Design review of the part built by this model. Coordinates are the model's own, in mm. Face numbers are marked on the shaded views. A direction names the side the tool comes from. Coordinates: 2 decimals unless noted, no trailing zeros. Write each loop counter-clockwise with the first axis right and the second up, starting at its lowest first coordinate (ties: lowest second). Pieces come first, ordered by that corner, then holes. Notation, with made-up numbers: (61.25, -3.5) -> (110.25, -3.5) arc R27 ccw to (110.25, 17.5) -> close; hole circle Ø5 at (-24.75, -34.75). An arc over 180 degrees is marked (long way). Answer in a Markdown table with one row per item. Add a question column.
Item 1: Clearance check with flat-ended pins moving along their axes: P1, Ø12, axis at x = 18.5, y = -9.5, coming from the -Z side; P2, Ø8, axis at x = 15.5, z = 12.5, coming from the -Y side; P3, Ø6.5, axis at x = -19.5, y = -6, coming from the +Z side; P4, Ø12, axis at x = -2, y = -7.5, coming from the -Z side. State where each tip first meets the part, or that it passes through.
Item 2: Draft analysis for pull direction X (two halves, no side actions). For the marked faces 5, 6 and 7, state which applies: released by +X, released by -X, zero draft, split by the parting line, or undercut.
Item 3: For the marked faces 1, 2, 3 and 4, list the 3-axis set-ups (+Z, -Z, +X, -X, +Y, -Y) from which the entire face can be reached by the end or side of a thin tool; tool diameter is ignored.
Item 4: Take a section at D-D, the plane z = 20. Write out the cut boundary in (x, y), and give its area (3 significant figures).
Item 5: To check wall thickness, follow line 1 (Z direction, x = 17, y = -8.5); line 2 (X direction, y = -5.5, z = -15); line 3 (X direction, y = -13.5, z = -16). State the ranges of each line that lie inside material, in increasing order.
Item 6: Take a section at C-C, the plane z = -15.5. Write out the cut boundary in (x, y), and give its area (3 significant figures).
Item 7: Take a section at A-A, the plane y = -14. Write out the cut boundary in (x, z).
Item 8: Take a section at B-B, the plane y = -7.5. Give the number of separate pieces and of enclosed holes in the cut face, and give its area (3 significant figures).
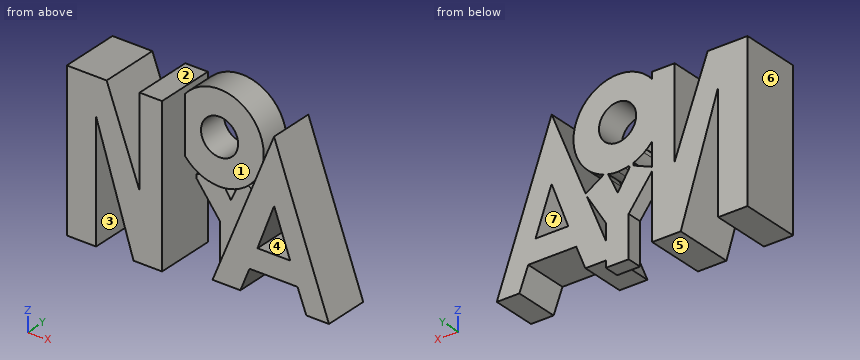
from build123d import *

# Parameters (mm, degrees)
F6_DEPTH  = 20
F7_DEPTH  = 5
F2_R      = 14.8981709713
F8_DEPTH  = 10
F9_DEPTH  = 15
F5_R      = 6.2195311323
F10_DEPTH = 20.001


with BuildPart() as f6:
    # F1 (on Front) → F6 (new body)
    with BuildSketch(Plane.XZ):
        Polygon((-29.4090751559, 23.7889681011), (-29.4090751559, -28.2321553677), (-19.5761136711, -28.2358180233), (-19.5761136711, 11.5612922236), (-7.0128426887, -28.2359085977), (2.5514548179, -28.2359085977), (2.5514548179, 23.8814018667), (-4.9865087494, 23.8814018667), (-4.9865087494, -6.1893938109), (-16.0414669663, 23.7889681011), align=None)
    extrude(amount=F6_DEPTH)



with BuildPart() as f7:
    # F3 (on Front) → F7 (new body)
    with BuildSketch(Plane.XZ):
        Polygon((10.5204042047, -2.2638426162), (8.7501741946, -1.767860345), (8.7501741946, -2.6882454621), (2.6086692233, -5.1982523873), (2.6086692233, -6.4965714701), (10.4526793584, -16.883123666), (10.4526793584, -30.7555552572), (18.1284062564, -30.7555552572), (18.1284062564, -16.9692430645), (24.9908941437, -5.8241511643), (18.8475046307, -2.0414155442), (18.2504130668, -1.177824098), (17.1879893938, -1.9123892853), (17.4144990742, -2.239997033), (14.0946339816, -9.1059375554), (10.1119214669, -2.7744469699), align=None)
    extrude(amount=F7_DEPTH)


with BuildPart() as f6_1:
    add(f6.part)

    add(f7.part)  # F8 merges F7
    # F2 (on Front) → F8 (join)
    with BuildSketch(Plane.XZ):
        with Locations((14.0610327944, 12.1286660433)):
            Circle(F2_R)
    extrude(amount=F8_DEPTH)

    # F4 (on Front) → F9 (join)
    with BuildSketch(Plane.XZ):
        Polygon((54.6711832285, -28.5867527127), (36.2575501204, 22.3937444389), (15.6466114905, -28.5145416856), (24.9638519287, -28.5145416856), (28.0255712569, -20.860247314), (44.1284738481, -20.860247314), (47.089099884, -28.5867527127), align=None)
    extrude(amount=F9_DEPTH)

    # F5 (on Front) + F0 (on Front) → F10 (cut, through all)
    with BuildSketch(Plane.XZ):
        Polygon((10.4725992623, -2.2513235357), (10.0927506823, -2.7248826654), (14.1619760543, -9.0967444703), (17.3306893557, -2.3522656411), (16.3500196487, -2.7850975748), (14.0968551859, -2.7850975748), (11.5571627393, -2.5246159639), align=None)
        with Locations((14.1619760543, 12.4046513811)):
            Circle(F5_R)
        Polygon((4.5241662301, 0.7314007962), (4.2605670169, 0.7808398308), (4.2605670169, -4.4249454513), (8.7323186063, -2.633718365), (8.7323186063, -1.8077495305), (7.9755438492, -1.6129313735), (6.1521744356, -0.636126264), align=None)
    with BuildSketch(Plane.XZ):
        Polygon((30.7015124708, -13.6729935011), (41.6589528322, -13.6729935011), (36.2836048007, 1.1847094047), align=None)
    extrude(amount=F10_DEPTH, mode=Mode.SUBTRACT)


solid = f6_1.part
Answers:
| question | item | result |
|---|---|---|
| 1 | P1 | stops at z = -30.76 |
| 1 | P2 | passes through |
| 1 | P3 | stops at z = 23.79 |
| 1 | P4 | stops at z = -28.24 |
| 2 | face 5 | zero draft |
| 2 | face 6 | released by -X |
| 2 | face 7 | undercut |
| 3 | face 1 | +Z, -Y |
| 3 | face 2 | +Z, -X, +Y, -Y |
| 3 | face 3 | -Z, +Y, -Y |
| 3 | face 4 | +Y, -Y |
| 4 | outline | (-29.41, -20) -> (-14.64, -20) -> (-14.64, 0) -> (-29.41, 0) -> close; (-4.99, -20) -> (2.55, -20) -> (2.55, -10) -> (26.71, -10) -> (26.71, 0) -> (-4.99, 0) -> close; (35.29, -15) -> (37.12, -15) -> (37.12, 0) -> (35.29, 0) -> close |
| 4 | area | 715 mm^2 |
| 5 | line 1 | z = -28.51 to -25.17, -2.48 to 6.87, 17.94 to 26.73 |
| 5 | line 2 | x = -29.41 to -19.58, -11.19 to 2.55, 21.12 to 49.76 |
| 5 | line 3 | x = -29.41 to -19.58, -10.88 to 2.55, 20.71 to 50.12 |
| 6 | outline | (-29.41, -20) -> (-19.58, -20) -> (-19.58, 0) -> (-29.41, 0) -> close; (-11.03, -20) -> (2.55, -20) -> (2.55, 0) -> (-11.03, 0) -> close; (9.41, -5) -> (19.03, -5) -> (19.03, 0) -> (9.41, 0) -> close; (20.92, -15) -> (49.94, -15) -> (49.94, 0) -> (20.92, 0) -> close |
| 6 | area | 952 mm^2 |
| 7 | outline | (-29.41, -28.23) -> (-19.58, -28.24) -> (-19.58, 11.56) -> (-7.01, -28.24) -> (2.55, -28.24) -> (2.55, 23.88) -> (-4.99, 23.88) -> (-4.99, -6.19) -> (-16.04, 23.79) -> (-29.41, 23.79) -> close; (15.65, -28.51) -> (24.96, -28.51) -> (28.03, -20.86) -> (44.13, -20.86) -> (47.09, -28.59) -> (54.67, -28.59) -> (36.26, 22.39) -> close; hole (30.7, -13.67) -> (41.66, -13.67) -> (36.28, 1.18) -> close |
| 8 | separate pieces | 2 |
| 8 | enclosed holes | 2 |
| 8 | area | 2,550 mm^2 |
